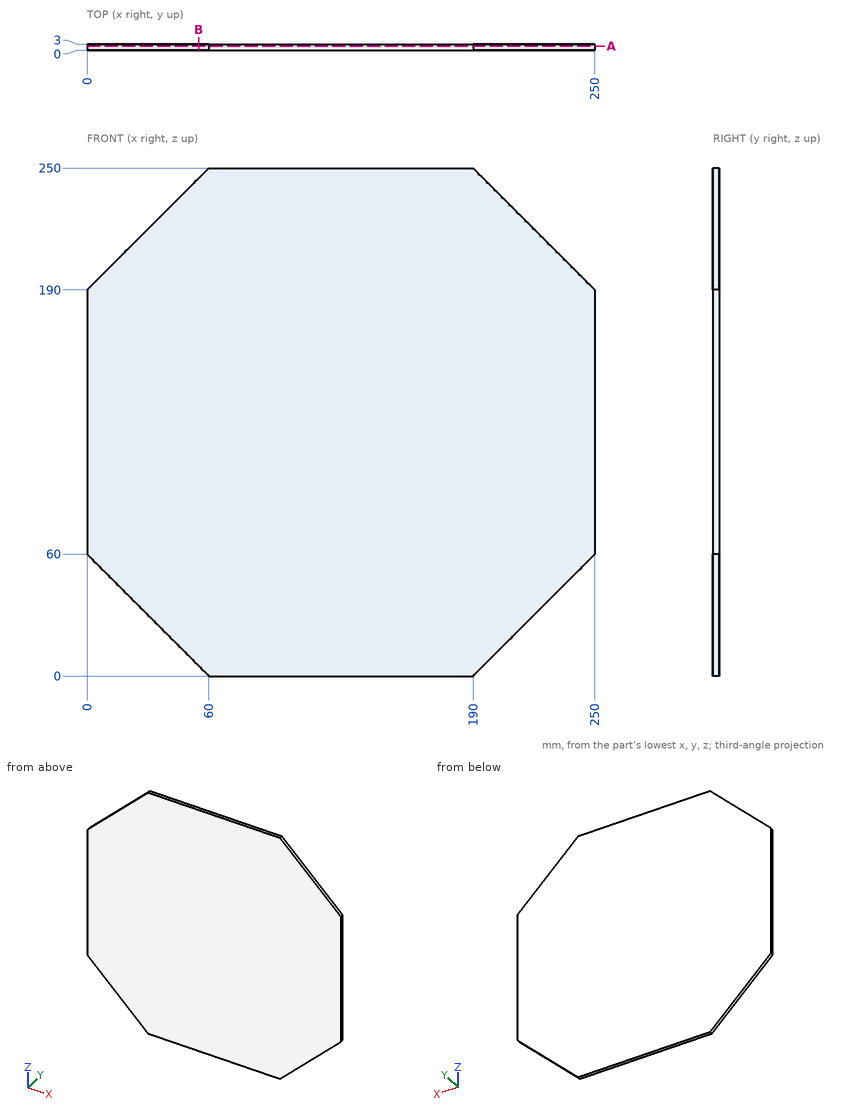
Design review of the part shown in the three views and the two pictorial views. Dimensions are in mm from the part's minimum x, y and z. Coordinates: 2 decimals unless noted, no trailing zeros. Order: outer loops, then holes, each group sorted by start corner. A loop starts at its lowest first (then second) coordinate and runs counter-clockwise, first axis right, second up. Notation, with made-up numbers: (54, 20.25) - (102, 20.25) arc R21 cw to (102, 45.25) - close; hole circle Ø8 at (-23, -35.75). An arc over 180 degrees is marked (long way). Answer as CSV lines item,"result". Start each with the question number.
1) Add section A-A (y = 2). State the section outline as (x, z) points.
2) To check wall thickness, follow line 1 along X through (y, z) = (2.2, 18.5); line 2 along X through (y, z) = (1.8, 224.5); line 3 along Z through (x, y) = (203, 2.95). State the ranges of each line that lie inside material, in increasing order. Write a range as [from, to].
3) Add section B-B (x = 55). State the section outline as (y, z) points, then the cut area to 3 significant figures.
Result:
1,outline,"(0, 60) - (60, 0) - (190, 0) - (250, 60) - (250, 190) - (190, 250) - (60, 250) - (0, 190) - close"
2,line 1,"[41.5, 208.5]"
2,line 2,"[34.5, 215.5]"
2,line 3,"[13, 237]"
3,outline,"(0, 5) - (3, 5) - (3, 245) - (0, 245) - close"
3,area,"720 mm^2"
